Geometry: final body of the model. Coordinates: model frame, mm. Round coordinates to 2 decimals unless told otherwise and drop trailing zeros. Order: outer loops, then holes, each group sorted by start corner. A loop starts at its lowest first (then second) coordinate and runs counter-clockwise, first axis right, second up. Notation, with made-up numbers: M 10,24.5 L 25,24.5 A33 ccw 25,61.5 Z; hole C 49,30.25 d7. An arc over 180 degrees is marked long. Return JSON: item names as keys, results as strings. Group by question number.
Q1. Cut plane B-B on x = 10. Output: boundary loops of the cut face in (y, z), and give its area (3 significant figures).
Q2. Cut plane D-D on z = 8.25. Output: boundary loops of the cut face in (x, y), and give its area (3 significant figures).
Q3. Ray query, probe 1 along Z at (x, y) = (10, -3.2); probe 2 along X at (y, z) = (-2.5, -1.75); probe 3 along Z at (x, y) = (8.5, -0.7). Return the intervals inside material, ascending.
Q4. Mould query, pull axis Z, two halves, no side actions, for faces 1 (the face through (7.46, -2.53, 1.05)), 2 (the face through (19.5, -2, 0)), 3 (the face through (18.64, -2.46, -8.6)). Classes: released by +Z, released by -Z, zero draft, split by the parting line, or undercut.
Q5. Cut plane A-A on z = 0. Output: boundary loops of the cut face in (x, y).
Q6. Cut plane C-C on y = -3.45. Output: boundary loops of the cut face in (x, z), and give its area (3 significant figures).
```python
from build123d import *

# Parameters (mm, degrees)
PROFILE_DEPTH = 5
M5_HOLE_D     = 5.5


with BuildPart() as part:
    # Profile Sketch → Profile (new body)
    with BuildSketch(Plane(origin=(0, 0, 0), x_dir=(1, 0, 0), z_dir=(0, 1, 0))):
        with BuildLine():
            Line((-16.5, -9.5), (16.5, -9.5))
            ThreePointArc((16.5, -9.5), (18.621320344, -8.621320344), (19.5, -6.5))
            Line((19.5, -6.5), (19.5, 6.5))
            ThreePointArc((19.5, 6.5), (18.621320344, 8.621320344), (16.5, 9.5))
            Line((16.5, 9.5), (-16.5, 9.5))
            ThreePointArc((-16.5, 9.5), (-18.621320344, 8.621320344), (-19.5, 6.5))
            Line((-19.5, 6.5), (-19.5, -6.5))
            ThreePointArc((-19.5, -6.5), (-18.621320344, -8.621320344), (-16.5, -9.5))
        make_face()
    extrude(amount=-PROFILE_DEPTH)

    # M5 Hole (through all)
    with Locations(Plane(origin=(0, 0, 0), x_dir=(1, 0, 0), z_dir=(0, 1, 0))):
        with Locations((10, 0)):
            Hole(M5_HOLE_D / 2)


solid = part.part
```
Result sheet:
{
 "1": {"outline": "M -5,-9.5 L 0,-9.5 L 0,-2.75 L -5,-2.75 Z; M -5,2.75 L 0,2.75 L 0,9.5 L -5,9.5 Z", "area": "67.5 mm²"},
 "2": {"outline": "M -18.94,-5 L 18.94,-5 L 18.94,0 L -18.94,0 Z", "area": "189 mm²"},
 "3": {"probe 1": "z = -9.5 to -2.75, 2.75 to 9.5", "probe 2": "x = -19.5 to 7.88, 12.12 to 19.5", "probe 3": "z = -9.5 to -2.3, 2.3 to 9.5"},
 "4": {"face 1": "undercut", "face 2": "zero draft", "face 3": "released by -Z"},
 "5": {"outline": "M -19.5,-5 L 7.25,-5 L 7.25,0 L -19.5,0 Z; M 12.75,-5 L 19.5,-5 L 19.5,0 L 12.75,0 Z"},
 "6": {"outline": "M -19.5,-6.5 A3 ccw -16.5,-9.5 L 16.5,-9.5 A3 ccw 19.5,-6.5 L 19.5,6.5 A3 ccw 16.5,9.5 L -16.5,9.5 A3 ccw -19.5,6.5 Z; hole C 10,0 d5.5", "area": "710 mm²"}
}
